Geometry: final body of the model. Coordinates: model frame, mm. A direction names the side the tool comes from. Round coordinates to 2 decimals unless told otherwise and drop trailing zeros. Loops run counter-clockwise (first coordinate to the right, second up) from the corner with the lowest first, then second, coordinate; pieces in that order, holes last. Notation, with made-up numbers: (84.25, 49.5) -> (97.25, 49.5) arc R25 cw to (97.25, 80.5) -> close; hole circle Ø2 at (33, -2.5). An arc over 180 degrees is marked (long way). Answer in a Markdown table with one row per item.
```python
from build123d import *

# Parameters (mm, degrees)
SKETCH1_W           = 20.32
SKETCH1_H           = 10.16
BOSS_EXTRUDE1_DEPTH = 29.21
SKETCH1_4_W         = 20.32
SKETCH1_4_H         = 10.16
BOSS_EXTRUDE2_DEPTH = 29.21
SKETCH5_W           = 3.048
SKETCH5_H           = 40.64
BOSS_EXTRUDE4_DEPTH = 58.42
SKETCH10_W          = 39.323622634
SKETCH10_H          = 20.32
CUT_EXTRUDE2_DEPTH  = 101.12884899
CUT_EXTRUDE4_START  = -40.64
CUT_EXTRUDE4_DEPTH  = 40.64
CUT_EXTRUDE5_REACH  = 95.3
SKETCH13_W          = 20.066
SKETCH13_H          = 39.878


# Read off the part's stored shape, not the designer's step: Cut-Extrude4
with BuildPart() as part:
    # Sketch1 → Boss-Extrude1 (new, symmetric)
    with BuildSketch(Plane.XY):
        with Locations((-10.16, 15.24)):
            Rectangle(SKETCH1_W, SKETCH1_H)
    boss_extrude1 = extrude(amount=BOSS_EXTRUDE1_DEPTH, both=True)

    # Mirror1: Boss-Extrude1 across plane
    add(boss_extrude1.mirror(Plane(origin=(0, 0, 0), x_dir=(0, 0, 1), z_dir=(1, 0, 0))))



with BuildPart() as body_2:
    # Sketch1_4 → Boss-Extrude2 (new, symmetric)
    with BuildSketch(Plane.XY):
        with Locations((-10.16, -15.24)):
            Rectangle(SKETCH1_4_W, SKETCH1_4_H)
        with Locations((10.16, -15.24)):
            Rectangle(SKETCH1_4_W, SKETCH1_4_H)
    extrude(amount=BOSS_EXTRUDE2_DEPTH, both=True)


with BuildPart() as part_1:
    add(part.part)

    add(body_2.part)  # Boss-Extrude4 merges body 2
    # Sketch5 → Boss-Extrude4 (add)
    with BuildSketch(Plane(origin=(20.32, 0, 0), x_dir=(0, 0, -1), z_dir=(1, 0, 0))):
        with Locations((-27.686, 0)):
            Rectangle(SKETCH5_W, SKETCH5_H)
        with Locations((27.686, 0)):
            Rectangle(SKETCH5_W, SKETCH5_H)
    extrude(amount=BOSS_EXTRUDE4_DEPTH)

    # Sketch8 → CBORE for M1.6 SHCS1 (revolve, cut)
    with BuildSketch(Plane(origin=(-16.51, 20.32, 0), x_dir=(0, 0, 1), z_dir=(1, 0, 0))):
        Polygon((0, 0), (0, 40.64), (0.9, 40.64), (0.9, 1.6), (1.75, 1.6), (1.75, 0.025), (1.775, 0), align=None)
    revolve(axis=Axis((-16.51, 26.67, 0), (0, -1, 0)), mode=Mode.SUBTRACT)

    # Sketch10 → Cut-Extrude2 (cut, through all)
    with BuildSketch(Plane.XY.offset(29.21)):
        with Locations((59.078188683, 0)):
            Rectangle(SKETCH10_W, SKETCH10_H)
    extrude(amount=-CUT_EXTRUDE2_DEPTH, mode=Mode.SUBTRACT)

    # Cut-Extrude4 outline → Cut-Extrude4 (cut)
    with BuildSketch(Plane(origin=(0, 20.32, 0), x_dir=(1, 0, 0), z_dir=(0, 1, 0)).offset(CUT_EXTRUDE4_START)):
        with BuildLine():
            ThreePointArc((20.32, -29.21), (-4.704156829, -21.149913849), (-20.32, 0))
            Line((-20.32, 0), (-20.32, -29.21))
            Line((-20.32, -29.21), (20.32, -29.21))
        make_face()
        with BuildLine():
            ThreePointArc((-20.32, 0), (-4.704156829, 21.149913849), (20.32, 29.21))
            Line((20.32, 29.21), (-20.32, 29.21))
            Line((-20.32, 29.21), (-20.32, 0))
        make_face()
    extrude(amount=CUT_EXTRUDE4_DEPTH, mode=Mode.SUBTRACT)

    # Sketch13 → Cut-Extrude5 (cut, up to next)
    with BuildSketch(Plane(origin=(0, 20.32, 0), x_dir=(1, 0, 0), z_dir=(0, 1, 0)), mode=Mode.PRIVATE) as cut_extrude5_sk1:
        with Locations((6.985, 0)):
            Rectangle(SKETCH13_W, SKETCH13_H)
    cut_extrude5_tool1 = extrude(cut_extrude5_sk1.sketch, amount=-CUT_EXTRUDE5_REACH, mode=Mode.PRIVATE) & part_1.part
    add(cut_extrude5_tool1.solids().sort_by_distance((6.985, 20.32, 0))[0], mode=Mode.SUBTRACT)


solid = part_1.part
```
Item 1: Ray query, L1, parallel to X at y = 15, z = 0; L2, parallel to X at y = 19.25, z = 0; L3, parallel to X at y = -17.75, z = 0. Return the intervals inside material, ascending.
Ans:
| item | result |
|---|---|
| L1 | -20.32 to -17.41, -15.61 to -3.05, 17.02 to 20.32 |
| L2 | -20.32 to -18.26, -14.76 to -3.05, 17.02 to 20.32 |
| L3 | -20.32 to -17.41, -15.61 to 20.32 |
Item 2: Mould query, pull axis Y, two halves, no side actions, for faces 6 (the flat face through (59, -10.16, -28)), 7 (the cylindrical face through (-4.399, -15.311, 21.367)), 8 (the flat face through (18, 20.32, 2)), 9 (the flat face through (7, -20.32, 7)). Classes: released by +Y, released by -Y, zero draft, split by the parting line, or undercut.
Ans:
| item | result |
|---|---|
| face 6 | undercut |
| face 7 | zero draft |
| face 8 | released by +Y |
| face 9 | released by -Y |
Item 3: Set-up query: faces 1 (the flat face through (59, -10.16, 28)), 2 (the flat face through (78.74, -15, -28)), 3 (the flat face through (20.32, 15, 0)), 4 (the flat face through (7, 15, -19.939)), 5 (the flat face through (36, 0, -29.21)). Return all of +Z, -Z, +X, -X, +Y, -Y with unobstructed straight access to the full face (end or side cutting, diameter ignored); none if empty.
Ans:
| item | result |
|---|---|
| face 1 | +Z, -Z, +X |
| face 2 | +Z, -Z, +X, +Y, -Y |
| face 3 | +X, +Y, -Y |
| face 4 | +Y |
| face 5 | -Z, +X, -X, +Y, -Y |
Item 4: Section query D-D, the plane z = 5. Output: boundary loops of the cut face in (x, y), and give its area (3 significant figures).
Ans:
| item | result |
|---|---|
| outline | (-18.28, -20.32) -> (20.32, -20.32) -> (20.32, -10.16) -> (-18.28, -10.16) -> close; (-18.28, 10.16) -> (-3.05, 10.16) -> (-3.05, 20.32) -> (-18.28, 20.32) -> close; (17.02, 10.16) -> (20.32, 10.16) -> (20.32, 20.32) -> (17.02, 20.32) -> close |
| area | 580 mm2 |
Item 5: Section query C-C, the plane y = 15. Output: boundary loops of the cut face in (x, z), and give its area (3 significant figures).
Ans:
| item | result |
|---|---|
| outline | (-20.32, 0) arc R42.88 ccw to (20.32, -29.21) -> (78.74, -29.21) -> (78.74, -26.16) -> (20.32, -26.16) -> (20.32, 26.16) -> (78.74, 26.16) -> (78.74, 29.21) -> (20.32, 29.21) arc R42.88 ccw to start; hole circle Ø1.8 at (-16.51, 0); hole (-3.05, -19.94) -> (17.02, -19.94) -> (17.02, 19.94) -> (-3.05, 19.94) -> close |
| area | 1,290 mm2 |
Item 6: Section query B-B, the plane y = -3. Output: boundary loops of the cut face in (x, z), and give its area (3 significant figures).
Ans:
| item | result |
|---|---|
| outline | (20.32, -29.21) -> (39.42, -29.21) -> (39.42, -26.16) -> (20.32, -26.16) -> close; (20.32, 26.16) -> (39.42, 26.16) -> (39.42, 29.21) -> (20.32, 29.21) -> close |
| area | 116 mm2 |
Item 7: First-contact query: P1, Ø5, axis at x = -3, y = 12, coming from the +Z side; P2, Ø0.9, axis at y = -3.5, z = -27.5, coming from the -X side; P3, Ø3, axis at x = -16.51, z = 0, coming from the -Y side; P4, Ø8, axis at y = -14.5, z = -11, coming from the +X side. Flat tips, straight axial feed; report the tip coordinate or a pass-through.
Ans:
| item | result |
|---|---|
| P1 | z = 23.82 |
| P2 | x = 20.32 |
| P3 | y = -20.32 |
| P4 | x = 20.32 |
Item 8: Section query A-A, the plane x = 62. Output: boundary loops of the cut face in (y, z), and give its area (3 significant figures).
Ans:
| item | result |
|---|---|
| outline | (-20.32, -29.21) -> (-10.16, -29.21) -> (-10.16, -26.16) -> (-20.32, -26.16) -> close; (-20.32, 26.16) -> (-10.16, 26.16) -> (-10.16, 29.21) -> (-20.32, 29.21) -> close; (10.16, -29.21) -> (20.32, -29.21) -> (20.32, -26.16) -> (10.16, -26.16) -> close; (10.16, 26.16) -> (20.32, 26.16) -> (20.32, 29.21) -> (10.16, 29.21) -> close |
| area | 124 mm2 |
